```python
from build123d import *

# Parameters (mm, degrees)
ESBO_O1_R                = 3.325
RESSALTO_EXTRUS_O1_DEPTH = 4.7625


with BuildPart() as part:
    # Esboço1 → Ressalto-extrusão1 (new body)
    with BuildSketch(Plane.XY):
        with BuildLine():
            Line((-7.5, 0), (-7.5, 120))
            ThreePointArc((-7.5, 120), (0, 127.5), (7.5, 120))
            Line((7.5, 120), (7.5, 0))
            ThreePointArc((7.5, 0), (0, -7.5), (-7.5, 0))
        make_face()
        with Locations(Location((0, 120, 0), (0, 0, 180))):
            Circle(ESBO_O1_R, mode=Mode.SUBTRACT)
        with BuildLine():
            Line((2.246839856, -0.491640786), (0.697646517, 2.191640786))
            ThreePointArc((0.697646517, 2.191640786), (0, 2.3), (-0.697646517, 2.191640786))
            Line((-0.697646517, 2.191640786), (-2.246839856, -0.491640786))
            ThreePointArc((-2.246839856, -0.491640786), (-1.991858429, -1.15), (-1.549193338, -1.7))
            Line((-1.549193338, -1.7), (1.549193338, -1.7))
            ThreePointArc((1.549193338, -1.7), (1.991858429, -1.15), (2.246839856, -0.491640786))
        make_face(mode=Mode.SUBTRACT)
    extrude(amount=RESSALTO_EXTRUS_O1_DEPTH)


solid = part.part
```
Build history of the part. All positions in model axes, mm. A direction names the side the tool comes from. Round coordinates to 2 decimals unless told otherwise and drop trailing zeros. Order: outer loops, then holes, each group sorted by start corner. A loop starts at its lowest first (then second) coordinate and runs counter-clockwise, first axis right, second up. Notation, with made-up numbers: (-30, 64.25) -> (-17, 64.25) arc R24 cw to (-17, 86.25) -> close; hole circle Ø2 at (-33, 62.5). An arc over 180 degrees is marked (long way). Answer in a Markdown table with one row per item.
1) Band-saw the part on A-A on z = 1.7. Give the cut face in (x, y) (3 decimals), and give its area (3 significant figures).
Values:
| item | result |
|---|---|
| outline | (-7.5, 0) arc R7.5 ccw to (7.5, 0) -> (7.5, 120) arc R7.5 ccw to (-7.5, 120) -> close; hole circle Ø6.65 at (0, 120); hole (-2.247, -0.492) arc R2.3 ccw to (-1.549, -1.7) -> (1.549, -1.7) arc R2.3 ccw to (2.247, -0.492) -> (0.698, 2.192) arc R2.3 ccw to (-0.698, 2.192) -> close |
| area | 1,930 mm2 |
2) Which spindle directions (+Z, -Z, +X, -X, +Y, -Y) get a long thin tool onto all of the face, cutting with end or side? Do faces 1 (the flat face through (-1.46, 0.87, 2.35)), 2 (the flat face through (0, 61, 4.762)). Say none if no direction does.
Values:
| item | result |
|---|---|
| face 1 | +Z, -Z |
| face 2 | +Z, +X, -X, +Y, -Y |
3) Wall check: L1, parallel to Y at x = 0, z = 2.3 (3 decimals); L2, parallel to X at y = 120, z = 1.75 (3 decimals); L3, parallel to Y at x = 1.5, z = 2.35. Give the ranges that are in metal, low to high.
Values:
| item | result |
|---|---|
| L1 | -7.5 to -1.7, 2.3 to 116.675, 123.325 to 127.5 |
| L2 | -7.5 to -3.325, 3.325 to 7.5 |
| L3 | -7.35 to -1.7, 0.8 to 117.03, 122.97 to 127.35 |
4) Band-saw the part on B-B on x = -5. Give the cut face in (y, z).
Values:
| item | result |
|---|---|
| outline | (-5.59, 0) -> (125.59, 0) -> (125.59, 4.76) -> (-5.59, 4.76) -> close |
5) Pin check, flat tips, straight feed: P1, Ø1.5, axis at x = 2, z = 0.5, coming from the -Y side; P2, Ø1, axis at x = -1, z = 1.5, coming from the -Y side. Stop position of each tip, or through.
Values:
| item | result |
|---|---|
| P1 | y = -7.4 |
| P2 | y = -7.48 |
6) Mould opens along Y. For faces 3 (the flat face through (0, -1.7, 2)), 4 (the cylindrical face through (-0.16, 127.5, 2.35)), 5 (the flat face through (0, 61, 0)) say: released by +Y, released by -Y, zero draft, split by the parting line, or undercut.
Values:
| item | result |
|---|---|
| face 3 | undercut |
| face 4 | released by +Y |
| face 5 | zero draft |
